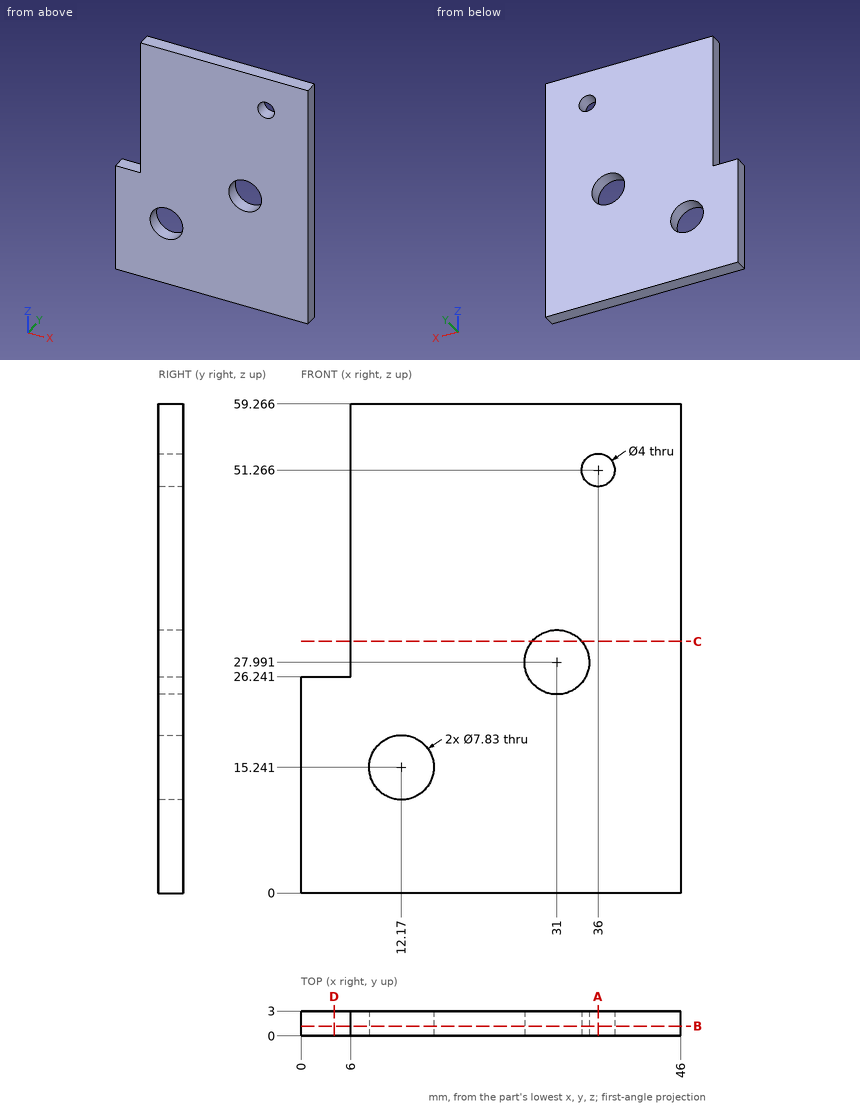
Print and shaded views of the part. All mm, measured from the part's lowest x, y and z. Give positions to 0.01 mm unless a question says otherwise; leave off trailing zeros. Loops run counter-clockwise (first coordinate to the right, second up) from the corner with the lowest first, then second, coordinate; pieces in that order, holes last. Notation, with made-up numbers: (-1.75, 89.25) -> (52.25, 89.25) arc R28 cw to (52.25, 118.25) -> close; hole circle Ø10 at (20.5, 39.25). An arc over 180 degrees is marked (long way). Use a Markdown table: item, result.
1. Slice it at C-C (z = 30.5). List the corners of the cut face in (x, y) (1 decimal), plus the area to 3 significant figures.
Check result:
| item | result |
|---|---|
| outline | (6, 0) -> (28, 0) -> (28, 3) -> (6, 3) -> close; (34, 0) -> (46, 0) -> (46, 3) -> (34, 3) -> close |
| area | 102 mm^2 |
2. Wall check: L1, parallel to X at y = 1.95, z = 33; L2, parallel to X at y = 0.2, z = 30.5 (1 decimal); L3, parallel to X at y = 0.2, z = 18.5 (1 decimal). Give the ranges that are in metal, low to high. Write a range as [from, to].
Check result:
| item | result |
|---|---|
| L1 | x = [6, 46] |
| L2 | x = [6, 28], [34, 46] |
| L3 | x = [0, 10], [14.3, 46] |
3. Slice it at B-B (y = 1.2). List the corners of the cut face in (x, z) (1 decimal).
Check result:
| item | result |
|---|---|
| outline | (0, 0) -> (46, 0) -> (46, 59.3) -> (6, 59.3) -> (6, 26.2) -> (0, 26.2) -> close; hole circle Ø7.8 at (12.2, 15.2); hole circle Ø7.8 at (31, 28); hole circle Ø4 at (36, 51.3) |
4. Slice it at A-A (x = 36). List the corners of the cut face in (y, z) (1 decimal), plus the area to 3 significant figures.
Check result:
| item | result |
|---|---|
| outline | (0, 0) -> (3, 0) -> (3, 49.3) -> (0, 49.3) -> close; (0, 53.3) -> (3, 53.3) -> (3, 59.3) -> (0, 59.3) -> close |
| area | 166 mm^2 |
5. Slice it at D-D (x = 4). List the corners of the cut face in (y, z).
Check result:
| item | result |
|---|---|
| outline | (0, 0) -> (3, 0) -> (3, 26.24) -> (0, 26.24) -> close |
